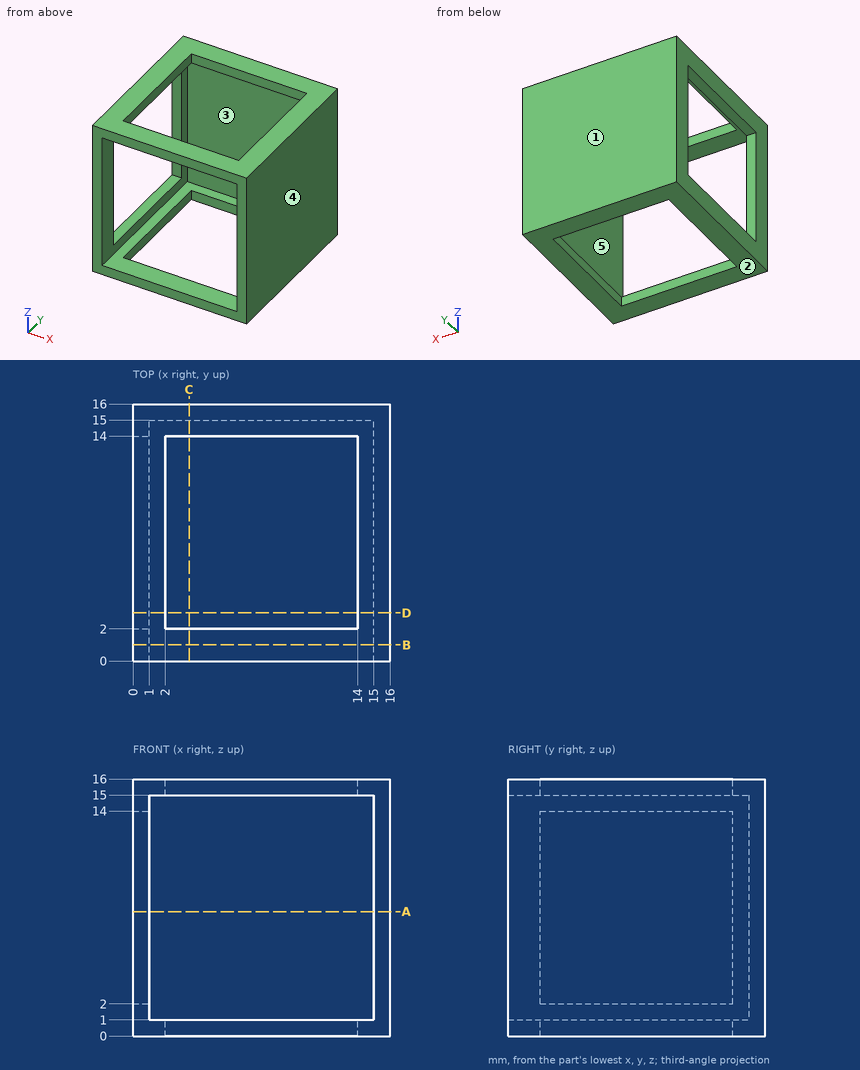
Here's the drawing with two shaded views (mm, measured from the low corner). I have some questions. A direction names the side the tool comes from. Round coordinates to 2 decimals unless told otherwise and drop trailing zeros. Order: outer loops, then holes, each group sorted by start corner. A loop starts at its lowest first (then second) coordinate and runs counter-clockwise, first axis right, second up. Notation, with made-up numbers: (10.5, 61) -> (26.5, 61) arc R36 ccw to (26.5, 95) -> close; hole circle Ø4 at (25.5, -15). An arc over 180 degrees is marked (long way). Use a Markdown table: item, result. Add a question column.
(1) Suppose I cut it at A-A, the plane z = 7.75. Please give me the cut outline in (x, y), and give its area (3 significant figures).
(2) I need wall thicknesses on line 1 along Z through (x, y) = (1.25, 4.5); line 2 along Y through (x, z) = (9.75, 12). Which ranges of each line are inside material? Lowest first, please.
(3) Suppose I cut it at B-B, the plane y = 1. Please give me the cut outline in (x, z), and give its area (3 significant figures).
(4) Suppose I cut it at C-C, the plane x = 3.5. Please give me the cut outline in (y, z).
(5) If we mould it in two halves opening along Z, with no side actions, what happens to the marked faces 1, 2 and 3? For each: released by +Z, released by -Z, zero draft, split by the parting line, or undercut.
(6) For pin 1 Ø4 at (x, z) = (8, 5) entering from -Y; pin 2 Ø0.8 at (x, y) = (0.5, 6) entering from -Z; pin 3 Ø8 at (y, z) = (9, 9.5) entering from -X, each with a flat end and sliding along its axis, tell me the tip position at first contact or that it passes through.
(7) Suppose I cut it at D-D, the plane y = 3. Please give me the cut outline in (x, z).
(8) For the marked faces 4 and 5, which set-ups out of +Z, -Z, +X, -X, +Y, -Y let a thin tool reach every point of the face, with its end or its side?
Verdict:
| question | item | result |
|---|---|---|
| 1 | outline | (0, 0) -> (1, 0) -> (1, 2) -> (0, 2) -> close; (0, 14) -> (1, 14) -> (1, 15) -> (15, 15) -> (15, 0) -> (16, 0) -> (16, 16) -> (0, 16) -> close |
| 1 | area | 34.0 mm2 |
| 2 | line 1 | 0 to 1, 15 to 16 |
| 2 | line 2 | 15 to 16 |
| 3 | outline | (0, 0) -> (16, 0) -> (16, 16) -> (0, 16) -> close; hole (1, 1) -> (15, 1) -> (15, 15) -> (1, 15) -> close |
| 3 | area | 60.0 mm2 |
| 4 | outline | (0, 0) -> (2, 0) -> (2, 1) -> (0, 1) -> close; (0, 15) -> (2, 15) -> (2, 16) -> (0, 16) -> close; (14, 0) -> (16, 0) -> (16, 16) -> (14, 16) -> (14, 15) -> (15, 15) -> (15, 1) -> (14, 1) -> close |
| 5 | face 1 | zero draft |
| 5 | face 2 | released by -Z |
| 5 | face 3 | undercut |
| 6 | pin 1 | y = 15 |
| 6 | pin 2 | z = 0 |
| 6 | pin 3 | x = 15 |
| 7 | outline | (0, 0) -> (2, 0) -> (2, 1) -> (1, 1) -> (1, 2) -> (0, 2) -> close; (0, 14) -> (1, 14) -> (1, 15) -> (2, 15) -> (2, 16) -> (0, 16) -> close; (14, 0) -> (16, 0) -> (16, 16) -> (14, 16) -> (14, 15) -> (15, 15) -> (15, 1) -> (14, 1) -> close |
| 8 | face 4 | +Z, -Z, +X, +Y, -Y |
| 8 | face 5 | -Y |
